Read the model definition and answer for the solid it produces. Units are mm, in the model's axes. A direction names the side the tool comes from. Coordinates: 2 decimals unless noted, no trailing zeros. Loops run counter-clockwise (first coordinate to the right, second up) from the corner with the lowest first, then second, coordinate; pieces in that order, holes last.
Q1. Straight lines are drawn through the part: line 1 (X direction, y = 361.5, z = 4); line 2 (Y direction, x = 111, z = 3); line 3 (X direction, y = 230, z = 2). For each, find the intervals that lie inside material, in ascending order.
Q2. Section B-B (y = 288) is taken. Give the vertices of the cut face in (x, z), then the cut area to 3 significant figures.
Q3. The mould has two halves that part along X. Classify faces 3 (the face through (-509.8, 323, 10)), 4 (the face through (-46, 327, 20)), 5 (the face through (-201, 435, 10)), 6 (the face through (176, 220, 10)): pulls with the +X half, pulls with the -X half, needs draft (parallel to the pull), parting line crosses it, or undercut.
Q4. Section C-C (z = 6.25) is taken. Give the vertices of the cut face in (x, y).
Q5. Which of the six approach directions +Z, -Z, +X, -X, +Y, -Y give full straight-line access (tool end or side, diameter ignored) to faces 1 (the face through (-33, 472.5, 10)), 2 (the face through (-275, 344, 10))?
Q6. Section A-A (x = 153) is taken. Give the vertices of the cut face in (y, z).
from build123d import *

# Parameters (mm, degrees)
CROQUIS1_W              = 1200
CROQUIS1_H              = 950
SALIENTE_EXTRUIR1_DEPTH = 20
CROQUIS2_W              = 150
CROQUIS2_H              = 180
CORTAR_EXTRUIR1_DEPTH   = 20
CROQUIS3_W              = 650
CROQUIS3_H              = 500
CORTAR_EXTRUIR2_DEPTH   = 20
CORTAR_EXTRUIR4_DEPTH   = 50
CROQUIS7_W              = 150
CROQUIS7_H              = 210
CORTAR_EXTRUIR5_DEPTH   = 50
CROQUIS8_W              = 1514.751276537
CROQUIS8_H              = 489.569354176
CORTAR_EXTRUIR6_DEPTH   = 30
CROQUIS9_W              = 1728.554056326
CROQUIS9_H              = 479.757846805
CORTAR_EXTRUIR7_DEPTH   = 30
CROQUIS10_W             = 90.2
CROQUIS10_H             = 295
CROQUIS10_W_2           = 170
CORTAR_EXTRUIR8_DEPTH   = 30


with BuildPart() as part:
    # Croquis1 → Saliente-Extruir1 (new body)
    with BuildSketch(Plane.XY):
        Rectangle(CROQUIS1_W, CROQUIS1_H)
    extrude(amount=SALIENTE_EXTRUIR1_DEPTH)

    # Croquis2 → Cortar-Extruir1 (cut)
    with BuildSketch(Plane.XY.offset(20)):
        with Locations((-200, 345)):
            Rectangle(CROQUIS2_W, CROQUIS2_H)
    extrude(amount=-CORTAR_EXTRUIR1_DEPTH, mode=Mode.SUBTRACT)

    # Croquis3 → Cortar-Extruir2 (cut)
    with BuildSketch(Plane(origin=(0, 0, 0), x_dir=(-1, 0, 0), z_dir=(0, 0, -1))):
        with Locations((-50, -165)):
            Rectangle(CROQUIS3_W, CROQUIS3_H)
    extrude(amount=-CORTAR_EXTRUIR2_DEPTH, mode=Mode.SUBTRACT)

    # Croquis6 → Cortar-Extruir4 (cut)
    with BuildSketch(Plane(origin=(0, 0, 0), x_dir=(-1, 0, 0), z_dir=(0, 0, -1))):
        Polygon((600, 175), (-600, 175), (-633.284588691, 175), (-633.284588691, -516.156085413), (737.025481355, -516.156085413), (737.025481355, 175), align=None)
    extrude(amount=-CORTAR_EXTRUIR4_DEPTH, mode=Mode.SUBTRACT)

    # Croquis7 → Cortar-Extruir5 (cut)
    with BuildSketch(Plane(origin=(0, 0, 0), x_dir=(-1, 0, 0), z_dir=(0, 0, -1))):
        with Locations((-175, 325)):
            Rectangle(CROQUIS7_W, CROQUIS7_H)
    extrude(amount=-CORTAR_EXTRUIR5_DEPTH, mode=Mode.SUBTRACT)

    # Croquis8 → Cortar-Extruir6 (cut)
    with BuildSketch(Plane(origin=(0, 0, 0), x_dir=(-1, 0, 0), z_dir=(0, 0, -1))):
        with Locations((-63.357770541, 717.284677088)):
            Rectangle(CROQUIS8_W, CROQUIS8_H)
    extrude(amount=-CORTAR_EXTRUIR6_DEPTH, mode=Mode.SUBTRACT)

    # Croquis9 → Cortar-Extruir7 (cut)
    with BuildSketch(Plane(origin=(0, 0, 0), x_dir=(-1, 0, 0), z_dir=(0, 0, -1))):
        with Locations((-91.228936592, -62.378923403)):
            Rectangle(CROQUIS9_W, CROQUIS9_H)
    extrude(amount=-CORTAR_EXTRUIR7_DEPTH, mode=Mode.SUBTRACT)

    # Croquis10 → Cortar-Extruir8 (cut)
    with BuildSketch(Plane(origin=(0, 0, 0), x_dir=(-1, 0, 0), z_dir=(0, 0, -1))):
        with Locations((554.9, 325)):
            Rectangle(CROQUIS10_W, CROQUIS10_H)
        with Locations((-515, 325)):
            Rectangle(CROQUIS10_W_2, CROQUIS10_H)
    extrude(amount=-CORTAR_EXTRUIR8_DEPTH, mode=Mode.SUBTRACT)


solid = part.part
Numbers:
1. line 1: x = -509.8 to -275, -125 to 100, 250 to 430
1. line 2: y = 177.5 to 220, 430 to 472.5
1. line 3: x = -509.8 to 100, 250 to 430
2. outline: (-509.8, 0) - (-275, 0) - (-275, 20) - (-509.8, 20) - close; (-125, 0) - (100, 0) - (100, 20) - (-125, 20) - close; (250, 0) - (430, 0) - (430, 20) - (250, 20) - close
2. area: 12,800 mm2
3. face 3: pulls with the -X half
3. face 4: needs draft
3. face 5: undercut
3. face 6: undercut
4. outline: (-509.8, 177.5) - (430, 177.5) - (430, 472.5) - (-509.8, 472.5) - close; hole (-275, 255) - (-125, 255) - (-125, 435) - (-275, 435) - close; hole (100, 220) - (250, 220) - (250, 430) - (100, 430) - close
5. face 1: +Z, -Z, +X, -X, +Y
5. face 2: +Z, -Z
6. outline: (177.5, 0) - (220, 0) - (220, 20) - (177.5, 20) - close; (430, 0) - (472.5, 0) - (472.5, 20) - (430, 20) - close
